Source: three-view drawing plus pictorial views. Frame: mm from the lowest corner of the part. A direction names the side the tool comes from. Round coordinates to 2 decimals unless told otherwise and drop trailing zeros. Order: outer loops, then holes, each group sorted by start corner. A loop starts at its lowest first (then second) coordinate and runs counter-clockwise, first axis right, second up. Notation, with made-up numbers: (-14, 37.25) - (21, 37.25) arc R26 ccw to (21, 62.25) - close; hole circle Ø1 at (-22, 27.5). An arc over 180 degrees is marked (long way). One line per item, written item: value. Start each with the question number.
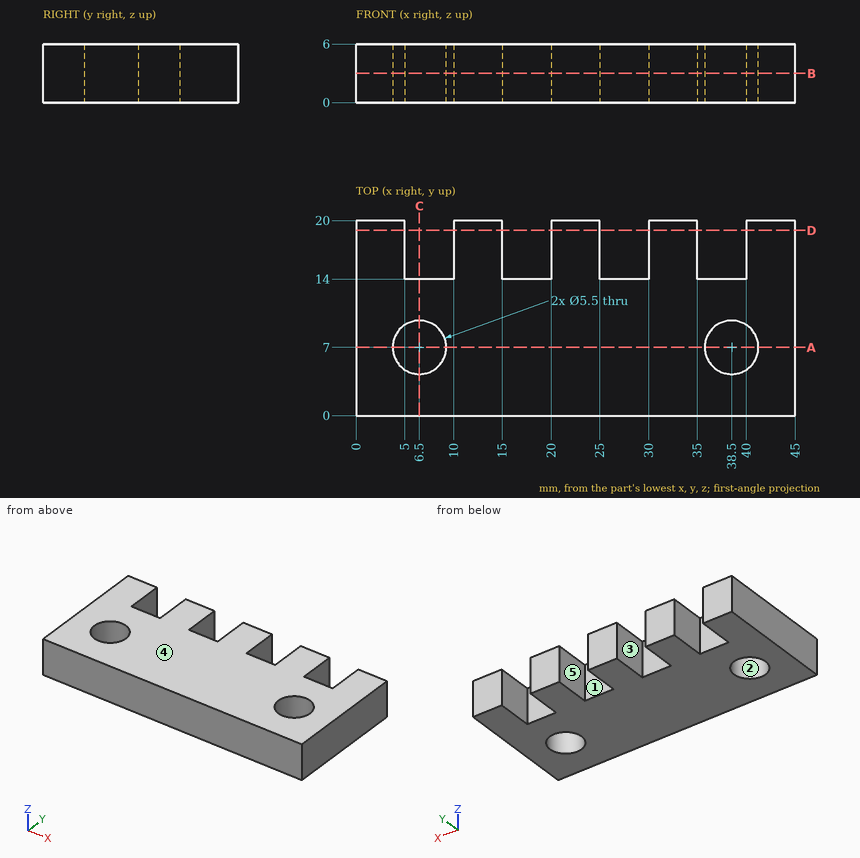
Item 1: First-contact query: pin 1 Ø1.5 at (x, z) = (16.5, 2) entering from +Y; pin 2 Ø3.5 at (x, y) = (38.5, 7) entering from -Z. Flat tips, straight axial feed; report the tip coordinate or a pass-through.
Item 2: Section query A-A on y = 7. Return loops of the section in (x, z), and give its area (3 significant figures).
Item 3: Pull-direction query (Y, two-part tool) for the marked faces 1, 2 and 3; classes: released by +Y, released by -Y, zero draft, split by the parting line, or undercut.
Item 4: Section query B-B on z = 3. Return loops of the section in (x, y), and give its area (3 significant figures).
Item 5: Line query: L1, parallel to X at y = 16.5, z = 4.9; L2, parallel to Y at x = 6.5, z = 2.2; L3, parallel to X at y = 6.25, z = 3.25. Output: solid intervals per line, ascending.
Item 6: Reachability of the marked faces 4 and 5 from +Z, -Z, +X, -X, +Y, -Y: full face, straight path, thin tool, end or side. Return the list, or none.
Item 7: Section query C-C on x = 6.5. Return loops of the section in (y, z).
Item 8: Section query D-D on y = 19. Return loops of the section in (x, z).
Geometry results:
1. pin 1: stops at y = 14
1. pin 2: passes through
2. outline: (0, 0) - (3.75, 0) - (3.75, 6) - (0, 6) - close; (9.25, 0) - (35.75, 0) - (35.75, 6) - (9.25, 6) - close; (41.25, 0) - (45, 0) - (45, 6) - (41.25, 6) - close
2. area: 204 mm^2
3. face 1: released by +Y
3. face 2: undercut
3. face 3: zero draft
4. outline: (0, 0) - (45, 0) - (45, 20) - (40, 20) - (40, 14) - (35, 14) - (35, 20) - (30, 20) - (30, 14) - (25, 14) - (25, 20) - (20, 20) - (20, 14) - (15, 14) - (15, 20) - (10, 20) - (10, 14) - (5, 14) - (5, 20) - (0, 20) - close; hole circle Ø5.5 at (6.5, 7); hole circle Ø5.5 at (38.5, 7)
4. area: 732 mm^2
5. L1: x = 0 to 5, 10 to 15, 20 to 25, 30 to 35, 40 to 45
5. L2: y = 0 to 4.25, 9.75 to 14
5. L3: x = 0 to 3.85, 9.15 to 35.85, 41.15 to 45
6. face 4: +Z, +X, -X, +Y, -Y
6. face 5: +Z, -Z, +Y
7. outline: (0, 0) - (4.25, 0) - (4.25, 6) - (0, 6) - close; (9.75, 0) - (14, 0) - (14, 6) - (9.75, 6) - close
8. outline: (0, 0) - (5, 0) - (5, 6) - (0, 6) - close; (10, 0) - (15, 0) - (15, 6) - (10, 6) - close; (20, 0) - (25, 0) - (25, 6) - (20, 6) - close; (30, 0) - (35, 0) - (35, 6) - (30, 6) - close; (40, 0) - (45, 0) - (45, 6) - (40, 6) - close
